The listing builds one solid part. Answer for the finished solid, in the listing's coordinates (mm). Face numbers are marked on the shaded views. A direction names the side the tool comes from. Give positions to 0.01 mm unless a question says otherwise; leave off trailing zeros. Order: outer loops, then holes, each group sorted by start corner. A loop starts at its lowest first (then second) coordinate and runs counter-clockwise, first axis right, second up. Notation, with made-up numbers: (37.5, 49.25) - (65.5, 49.25) arc R15 cw to (65.5, 63.25) - close; hole circle Ø2 at (71.5, 57.5). An arc over 180 degrees is marked (long way). Answer in a Markdown table with one row per item.
Autodesk Inventor part; units mm, degrees
ref_plane "YZ Plane" through (0, 0, 0) normal (1, 0, 0) x (0, 1, 0)
ref_plane "XZ Plane" through (0, 0, 0) normal (0, 1, 0) x (-1, 0, 0)
ref_plane "XY Plane" through (0, 0, 0) normal (0, 0, 1) x (1, 0, 0)
sketch "Sketch1" plane through (0, 0, 0) normal (0, 0, 1) x (1, 0, 0)
  circle A0 centre (0, 0) radius 2
  dimension "Diameter" = 4
extrude "Extrusion1" add sketch "Sketch1" along normal blind 6
sketch "Sketch2" plane through (0, 0, 6) normal (0, 0, 1) x (1, 0, 0)
  circle A0 centre (0, 0) radius 2
  circle A1 centre (0, 0) radius 3.5
  dimension "Head_Diameter" = 7
extrude "Extrusion2" add sketch "Sketch2" along normal blind 4 contours A0 | A1
sketch "Sketch3" plane through (0, 0, 10) normal (0, 0, 1) x (1, 0, 0)
  circle A0 centre (0, 0) radius 3.5
  circle A1 centre (0, 0) radius 1.7321 construction
  line L0 (0, 1.7321) -> (1.5, 0.866)
  line L1 (1.5, -0.866) -> (1.5, 0.866)
  line L2 (0, 1.7321) -> (-1.5, 0.866)
  line L3 (-1.5, -0.866) -> (-1.5, 0.866)
  line L4 (-1.5, -0.866) -> (0, -1.7321)
  line L5 (1.5, -0.866) -> (0, -1.7321)
  dimension "Hex_Width" = 3
extrude "Extrusion3" cut sketch "Sketch3" against normal blind 2 contours L0 L1 L5 L4 L3 L2
thread "Thread1"
chamfer "Chamfer1" distance 0.4 angle 45 2 edges at (-3.5, 0, 10) (-2, 0, 0)
equation "\"d9\" = ThreadLength"
equation "\"d12\" = Chamfer"
equation "\"ThreadLength\" = 6"
properties part number "SCREW,SOCKET HD,P,12.9,M4x0.7X6MM" material "Steel, MS"
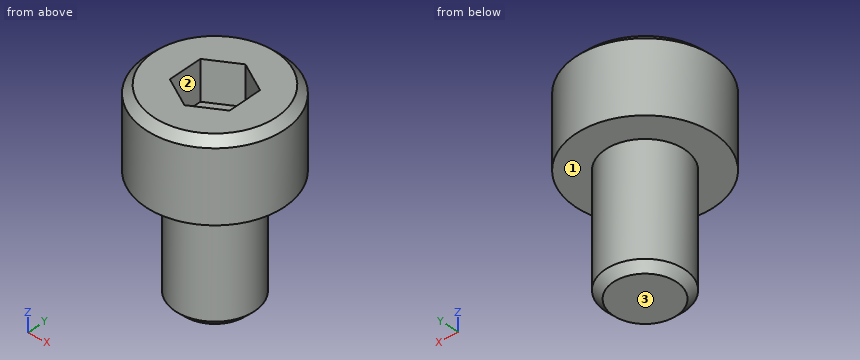
Item 1: Find section C-C on z = 4. Write down the section's boundary in (x, y).
Answer block:
| item | result |
|---|---|
| outline | circle Ø4 at (0, 0) |
Item 2: Which of the six approach directions +Z, -Z, +X, -X, +Y, -Y give full straight-line access (tool end or side, diameter ignored) to the marked faces 1, 2 and 3?
Answer block:
| item | result |
|---|---|
| face 1 | -Z |
| face 2 | +Z |
| face 3 | -Z, +X, -X, +Y, -Y |
Item 3: Consider line 1 (Z direction, x = -2.25, y = 2); line 2 (X direction, y = 1, z = 9); line 3 (Y direction, x = 1.25, z = 8.5). Determine where each line is inside the solid, lowest interval first.
Answer block:
| item | result |
|---|---|
| line 1 | 6 to 10 |
| line 2 | -3.35 to -1.27, 1.27 to 3.35 |
| line 3 | -3.27 to -1.01, 1.01 to 3.27 |
Item 4: Find section B-B on y = 0. Write down the section's boundary in (x, z), then the cut area to 3 significant figures.
Answer block:
| item | result |
|---|---|
| outline | (-3.5, 6) - (-2, 6) - (-2, 0.4) - (-1.6, 0) - (1.6, 0) - (2, 0.4) - (2, 6) - (3.5, 6) - (3.5, 9.6) - (3.1, 10) - (1.5, 10) - (1.5, 8) - (-1.5, 8) - (-1.5, 10) - (-3.1, 10) - (-3.5, 9.6) - close |
| area | 45.7 mm² |
Item 5: Each of these flat-tipped pins is pushed along its axis until it touches: P1, Ø0.5, axis at y = 0.5, z = 9, coming from the +X side; P2, Ø1.5, axis at x = 2.5, z = 4, coming from the +Y side. Where does it stop, or does it pass through?
Answer block:
| item | result |
|---|---|
| P1 | x = 3.49 |
| P2 | y = 0.97 |
Item 6: Find section A-A on z = 9. Write down the section's boundary in (x, y), then the cut area to 3 significant figures.
Answer block:
| item | result |
|---|---|
| outline | circle Ø7 at (0, 0); hole (-1.5, -0.87) - (0, -1.73) - (1.5, -0.87) - (1.5, 0.87) - (0, 1.73) - (-1.5, 0.87) - close |
| area | 30.7 mm² |
